Part model, mm, in its own coordinate system. Face numbers are marked on the shaded views. Round coordinates to 2 decimals unless told otherwise and drop trailing zeros. Loops run counter-clockwise (first coordinate to the right, second up) from the corner with the lowest first, then second, coordinate; pieces in that order, holes last. Notation, with made-up numbers: M 66.5,33 L 111.5,33 A26 ccw 111.5,59 Z; hole C -5,71.5 d5. An arc over 180 degrees is marked long. Write each question's results on one line, items separated by ' | '.
from build123d import *

# Parameters (mm, degrees)
F1_DEPTH = 6.35


with BuildPart() as f1:
    # F0 (on Top) → F1 (new body)
    with BuildSketch(Plane.XY):
        with BuildLine():
            Line((12.7, 19.05), (-12.7, 19.05))
            Line((-12.7, 19.05), (-12.7, 14.313342981))
            Line((-12.7, 14.313342981), (-8.89, 14.313342981))
            ThreePointArc((-8.89, 14.313342981), (-6.35, 16.853342981), (-3.81, 14.313342981))
            Line((-3.81, 14.313342981), (3.81, 14.313342981))
            ThreePointArc((3.81, 14.313342981), (6.35, 16.853342981), (8.89, 14.313342981))
            Line((8.89, 14.313342981), (12.7, 14.313342981))
            Line((12.7, 14.313342981), (12.7, 19.05))
        make_face()
        with BuildLine():
            Line((-8.89, 14.313342981), (-12.7, 14.313342981))
            Line((-12.7, 14.313342981), (-12.7, 9.525))
            Line((-12.7, 9.525), (12.7, 9.525))
            Line((12.7, 9.525), (12.7, 14.313342981))
            Line((12.7, 14.313342981), (8.89, 14.313342981))
            ThreePointArc((8.89, 14.313342981), (6.35, 11.773342981), (3.81, 14.313342981))
            Line((3.81, 14.313342981), (-3.81, 14.313342981))
            ThreePointArc((-3.81, 14.313342981), (-6.35, 11.773342981), (-8.89, 14.313342981))
        make_face()
        with BuildLine():
            Line((12.7, 9.525), (-12.7, 9.525))
            Line((-12.7, 9.525), (-12.7, 5.2324))
            Line((-12.7, 5.2324), (-7.1104125, 5.2324))
            ThreePointArc((-7.1104125, 5.2324), (-4.9276, 7.4152125), (-2.7447875, 5.2324))
            Line((-2.7447875, 5.2324), (2.7447875, 5.2324))
            ThreePointArc((2.7447875, 5.2324), (4.9276, 7.4152125), (7.1104125, 5.2324))
            Line((7.1104125, 5.2324), (12.7, 5.2324))
            Line((12.7, 5.2324), (12.7, 9.525))
        make_face()
        with BuildLine():
            Line((-7.1104125, 5.2324), (-12.7, 5.2324))
            Line((-12.7, 5.2324), (-12.7, 0))
            Line((-12.7, 0), (12.7, 0))
            Line((12.7, 0), (12.7, 5.2324))
            Line((12.7, 5.2324), (7.1104125, 5.2324))
            ThreePointArc((7.1104125, 5.2324), (4.9276, 3.0495875), (2.7447875, 5.2324))
            Line((2.7447875, 5.2324), (-2.7447875, 5.2324))
            ThreePointArc((-2.7447875, 5.2324), (-4.9276, 3.0495875), (-7.1104125, 5.2324))
        make_face()
    extrude(amount=F1_DEPTH)


solid = f1.part
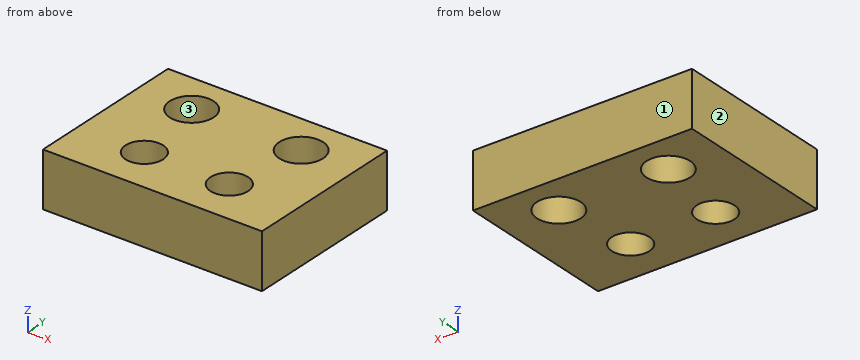
Item 1: Two-plate mould, pull along X, no slides. Class the marked faces 1, 2 and 3: +X half, -X half, draft (parallel to the pull), parting line (faces both ways), or undercut.
Filled sheet:
face 1: draft | face 2: -X half | face 3: undercut
Item 2: Band-saw the part on A-A on x = -6.35. Give the cut face in (y, z), and give its area (3 significant figures).
Filled sheet:
outline: M 0,0 L 3.58,0 L 3.58,6.35 L 0,6.35 Z; M 6.89,0 L 11.77,0 L 11.77,6.35 L 6.89,6.35 Z; M 16.85,0 L 19.05,0 L 19.05,6.35 L 16.85,6.35 Z | area: 67.7 mm^2
Item 3: Wall check: L1, parallel to Y at x = -6.35, z = 2.5; L2, parallel to Y at x = -4.5, z = 5.75; L3, parallel to X at y = 12.75, z = 5. Give the ranges that are in metal, low to high.
Filled sheet:
L1: 0 to 3.58, 6.89 to 11.77, 16.85 to 19.05 | L2: 0 to 3.09, 7.37 to 12.57, 16.05 to 19.05 | L3: -12.7 to -8.35, -4.35 to 4.35, 8.35 to 12.7
Item 4: Band-saw the part on C-C on x = 5.75. Give the cut face in (y, z), and give its area (3 significant figures).
Filled sheet:
outline: M 0,0 L 3.21,0 L 3.21,6.35 L 0,6.35 Z; M 7.25,0 L 11.85,0 L 11.85,6.35 L 7.25,6.35 Z; M 16.78,0 L 19.05,0 L 19.05,6.35 L 16.78,6.35 Z | area: 63.9 mm^2
Item 5: Band-saw the part on B-B on z = 0.75. Give the cut face in (x, y), and give its area (3 significant figures).
Filled sheet:
outline: M -12.7,0 L 12.7,0 L 12.7,19.05 L -12.7,19.05 Z; hole C -6.35,14.31 d5.08; hole C -4.93,5.23 d4.37; hole C 4.93,5.23 d4.37; hole C 6.35,14.31 d5.08 | area: 413 mm^2
Item 6: Drop a flat-ended pin along its axis: P1, Ø6, axis at x = 6.35, y = 14.31, coming from the -Z side. Give the stop position or say it passes through.
Filled sheet:
P1: z = 0
